Could you check a few things on this model? Use its own coordinates, in mm. A direction names the side the tool comes from. Give positions to 0.01 mm unless a question says otherwise; leave off trailing zeros. Write each loop counter-clockwise with the first axis right and the second up, starting at its lowest first coordinate (ties: lowest second). Pieces come first, ordered by that corner, then holes. Notation, with made-up numbers: (79.25, 87.25) - (90.25, 87.25) arc R25 cw to (90.25, 121.25) - close; hole circle Ø2 at (-28.5, 69). An arc over 180 degrees is marked (long way). Write item = value, one per line.
from build123d import *

# Parameters (mm, degrees)
F0_W     = 101.6
F0_H     = 279.4
F1_DEPTH = 19.05
F2_W     = 101.6
F2_H     = 12.7
F3_DEPTH = 2.54
F5_DEPTH = 25.4


with BuildPart() as f1:
    # F0 (on Front) → F1 (new body)
    with BuildSketch(Plane.XZ):
        with Locations((-78.7492649078, -32.640619709)):
            Rectangle(F0_W, F0_H)
    extrude(amount=F1_DEPTH)

    # F2 (on face) → F3 (join)
    with BuildSketch(Plane.XZ.offset(19.05)):
        with Locations((-78.7492649078, -115.190619709)):
            Rectangle(F2_W, F2_H)
        with Locations((-78.7492649078, -89.790619709)):
            Rectangle(F2_W, F2_H)
        with Locations((-78.7492649078, -64.390619709)):
            Rectangle(F2_W, F2_H)
        with Locations((-78.7492649078, -38.990619709)):
            Rectangle(F2_W, F2_H)
        with Locations((-78.7492649078, -13.590619709)):
            Rectangle(F2_W, F2_H)
        with Locations((-78.7492649078, 11.809380291)):
            Rectangle(F2_W, F2_H)
        with Locations((-78.7492649078, 37.209380291)):
            Rectangle(F2_W, F2_H)
        with Locations((-78.7492649078, 62.609380291)):
            Rectangle(F2_W, F2_H)
        with Locations((-78.7492649078, 88.009380291)):
            Rectangle(F2_W, F2_H)
        with Locations((-78.7492649078, -140.590619709)):
            Rectangle(F2_W, F2_H)
        with Locations((-78.7492649078, -165.990619709)):
            Rectangle(F2_W, F2_H)
    extrude(amount=F3_DEPTH)

    # F4 (on face) → F5 (cut)
    with BuildSketch(Plane.XZ.offset(19.05)):
        with BuildLine():
            Line((-86.6679660434, 81.659380291), (-70.8305637723, 81.659380291))
            ThreePointArc((-70.8305637723, 81.659380291), (-78.7492649078, 85.891007328), (-86.6679660434, 81.659380291))
        make_face()
        with BuildLine():
            ThreePointArc((-84.7382131406, 68.959380291), (-78.7492649078, 66.841007328), (-72.7603166751, 68.959380291))
            Line((-72.7603166751, 68.959380291), (-84.7382131406, 68.959380291))
        make_face()
        with BuildLine():
            ThreePointArc((-72.7603166751, 68.959380291), (-70.1536160982, 72.2622960149), (-69.2242649078, 76.366007328))
            ThreePointArc((-69.2242649078, 76.366007328), (-69.6346817216, 79.1318703655), (-70.8305637723, 81.659380291))
            Line((-70.8305637723, 81.659380291), (-86.6679660434, 81.659380291))
            ThreePointArc((-86.6679660434, 81.659380291), (-88.1661740472, 74.9351169543), (-84.7382131406, 68.959380291))
            Line((-84.7382131406, 68.959380291), (-72.7603166751, 68.959380291))
        make_face()
    extrude(amount=-F5_DEPTH, mode=Mode.SUBTRACT)


solid = f1.part
1. For pin 1 (10 mm diameter, centred on x = -86, z = 101.5, fed in from -Y); pin 2 (0.6 mm diameter, centred on x = -76.5, z = 68, fed in from +Y); pin 3 (0.8 mm diameter, centred on x = -64, y = -21, fed in from +Z), each with a flat end and sliding along its axis, tell me the tip position at first contact or that it passes through.
Filled sheet:
pin_1 = -19.05
pin_2 = -19.05
pin_3 = 94.36
2. Thinking about a two-plate mould opening in Z: for faces 3 (the face through (-79, -9, 107.059)), 4 (the face through (-79, -19.05, -26)), 5 (the face through (-129.549, -11, -35)), which applies, pulls with the +Z half, pulls with the -Z half, needs draft (parallel to the pull), parting line crosses it, or undercut?
Filled sheet:
face_3 = pulls with the +Z half
face_4 = undercut
face_5 = needs draft
3. I need wall thicknesses on line 1 (Y direction, x = -112, z = -27); line 2 (X direction, y = -16, z = 74). Which ranges of each line are inside material? Lowest first, please.
Filled sheet:
line_1 = -19.05 to 0
line_2 = -129.55 to -87.98, -69.52 to -27.95
4. Which directions (+Z, -Z, +X, -X, +Y, -Y) give clear straight access to the entire face, cutting with the end or side of a thin tool? Please do faces 1 (the face through (-79, -19.05, 25)), 2 (the face through (-79, -21.59, 12)).
Filled sheet:
face_1 = +X, -X, -Y
face_2 = +Z, -Z, +X, -X, -Y
5. If we section it at A-A, the plane z = -50: Please give me the cut outline in (x, y), and give its area (3 significant figures).
Filled sheet:
outline = (-129.55, -19.05) - (-27.95, -19.05) - (-27.95, 0) - (-129.55, 0) - close
area = 1,940 mm2
